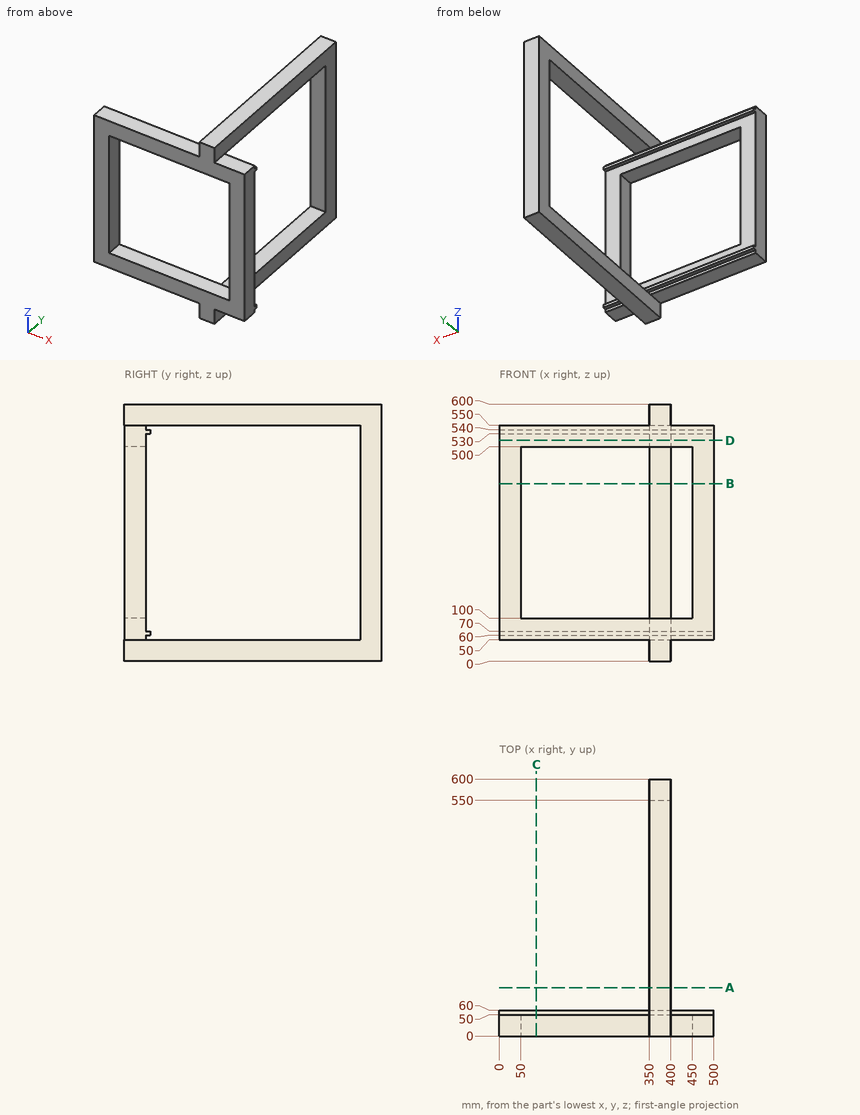
Verification items for this drawing (mm, ordinates from the low corner). Coordinates: 2 decimals unless noted, no trailing zeros. Order: outer loops, then holes, each group sorted by start corner. A loop starts at its lowest first (then second) coordinate and runs counter-clockwise, first axis right, second up. Notation, with made-up numbers: (69, -3) - (82, -3) arc R26 cw to (82, 13) - close; hole circle Ø9 at (-5.5, -7). An arc over 180 degrees is marked (long way). Answer as a JSON object with one key per item and string values. Group by question number.
Item 1: Sectioned sample at B-B, the plane z = 414. Record the cut outline in (x, y).
Item 2: Scan lines: probe 1 along Y at (x, z) = (361, 91); probe 2 along X at (y, z) = (556, 285); probe 3 along Y at (x, z) = (377.5, 444.5). Record each from-to range of solid material in increasing order.
Item 3: Sectioned sample at A-A, the plane y = 113. Record the cut outline in (x, z), and give its area (3 significant figures).
Item 4: Depth check by flat-ended pin: pin 1 Ø8 at (x, z) = (160, 64.5) entering from +Y; pin 2 Ø8 at (x, z) = (291.5, 546) entering from +Y; pin 3 Ø25 at (x, y) = (444, 31.5) entering from -Z; pin 4 Ø15 at (y, z) = (24, 326.5) entering from -X. Enter the tip coordinate at first touch or a pass-through.
Item 5: Sectioned sample at C-C, the plane x = 86. Record the cut outline in (y, z), and give its area (3 significant figures).
Item 6: Sectioned sample at D-D, the plane z = 515. Record the cut outline in (x, y), and give its area (3 significant figures).
Resolved:
{
 "1": {"outline": "(0, 0) - (50, 0) - (50, 50) - (0, 50) - close; (350, 550) - (400, 550) - (400, 600) - (350, 600) - close; (450, 0) - (500, 0) - (500, 50) - (450, 50) - close"},
 "2": {"probe 1": "0 to 50, 550 to 600", "probe 2": "350 to 400", "probe 3": "550 to 600"},
 "3": {"outline": "(350, 0) - (400, 0) - (400, 50) - (350, 50) - close; (350, 550) - (400, 550) - (400, 600) - (350, 600) - close", "area": "5,000 mm^2"},
 "4": {"pin 1": "y = 60", "pin 2": "y = 50", "pin 3": "z = 50", "pin 4": "x = 0"},
 "5": {"outline": "(0, 50) - (50, 50) - (50, 60) - (60, 60) - (60, 70) - (50, 70) - (50, 100) - (0, 100) - close; (0, 500) - (50, 500) - (50, 530) - (60, 530) - (60, 540) - (50, 540) - (50, 550) - (0, 550) - close", "area": "5,200 mm^2"},
 "6": {"outline": "(0, 0) - (500, 0) - (500, 50) - (0, 50) - close; (350, 550) - (400, 550) - (400, 600) - (350, 600) - close", "area": "27,500 mm^2"}
}
